from build123d import *

# Parameters (mm, degrees)
BOSS_EXTRUDE1_DEPTH     = 3
CUT_EXTRUDE1_DEPTH      = 67.166456759
CUT_EXTRUDE1_DEPTH_BACK = 67.166456759
SKETCH2_W               = 4.5
SKETCH2_H               = 4
SKETCH2_W_2             = 1.5
SKETCH2_W_3             = 6
VARFILLET1_START        = -1
VARFILLET1_DEPTH        = 5
BOSS_EXTRUDE2_START     = 1.8
SKETCH3_W               = 0.749988865
SKETCH3_H               = 2
SKETCH3_H_2             = 1.495913235
BOSS_EXTRUDE2_DEPTH     = 1.8


with BuildPart() as part:
    # Sketch1 → Boss-Extrude1 (new body)
    with BuildSketch(Plane.XY):
        with BuildLine():
            ThreePointArc((-34.616983549, 0), (-33.558491775, 0.00446614), (-32.5, 0))
            Line((-32.5, 0), (-32.5, 12))
            Line((-32.5, 12), (-48.75, 12))
            ThreePointArc((-48.75, 12), (-58.482695155, 8.177087189), (-65, 0))
            Line((-65, 0), (-34.616983549, 0))
        make_face()
        with BuildLine():
            ThreePointArc((-65, -4), (-49.931106105, -1.068651698), (-34.616983549, 0))
            Line((-34.616983549, 0), (-65, 0))
            Line((-65, 0), (-65, -4))
        make_face()
        with BuildLine():
            Line((-30.383016451, 0), (0, 0))
            ThreePointArc((0, 0), (-6.517304845, 8.177087189), (-16.25, 12))
            Line((-16.25, 12), (-32.5, 12))
            Line((-32.5, 12), (-32.5, 0))
            ThreePointArc((-32.5, 0), (-31.441508225, 0.00446614), (-30.383016451, 0))
        make_face()
        with BuildLine():
            Line((0, -4), (0, 0))
            Line((0, 0), (-30.383016451, 0))
            ThreePointArc((-30.383016451, 0), (-15.068893895, -1.068651698), (0, -4))
        make_face()
    extrude(amount=BOSS_EXTRUDE1_DEPTH)

    # Sketch2 → Cut-Extrude1 (cut, two sides: drawn at the far end of the back side and taken through both)
    with BuildSketch(Plane.XY.offset(3).offset(-CUT_EXTRUDE1_DEPTH_BACK)):
        with Locations((-34.75, 4)):
            Rectangle(SKETCH2_W, SKETCH2_H)
        with Locations((-31.75, 4)):
            Rectangle(SKETCH2_W_2, SKETCH2_H)
        with Locations((-28, 4)):
            Rectangle(SKETCH2_W_3, SKETCH2_H)
    extrude(amount=CUT_EXTRUDE1_DEPTH + CUT_EXTRUDE1_DEPTH_BACK, mode=Mode.SUBTRACT)

    # VarFillet1: read off the stored shape, not the designer's step
    # VarFillet1 outline → VarFillet1 (cut)
    with BuildSketch(Plane.XY.offset(VARFILLET1_START)):
        with BuildLine():
            ThreePointArc((-65, -4), (-64.073975757, -3.763989534), (-63.146180361, -3.535040754))
            add(Edge.make_bspline(
                [(-63.146180361, -3.535040754), (-65, -3.98501659), (-65, -2.07736738)],
                knots=[0, 0, 0, 1, 1, 1], degree=2, weights=[1, 0.61811012, 1]))
            Line((-65, -2.07736738), (-65, -4))
        make_face()
        with BuildLine():
            add(Edge.make_bspline(
                [(-0.135016199, 0.302883516), (0, 0.006564618), (0, -0.31906441)],
                knots=[0, 0, 0, 1, 1, 1], degree=2, weights=[1, 0.977238252, 1]))
            Line((0, -0.31906441), (0, 0))
            ThreePointArc((0, 0), (-0.066886569, 0.151718817), (-0.135016199, 0.302883516))
        make_face()
        with BuildLine():
            add(Edge.make_bspline(
                [(0, -2.07736738), (0, -3.98501659), (-1.853819639, -3.535040754)],
                knots=[0, 0, 0, 1, 1, 1], degree=2, weights=[1, 0.61811012, 1]))
            ThreePointArc((-1.853819639, -3.535040754), (-0.926024243, -3.763989534), (0, -4))
            Line((0, -4), (0, -2.07736738))
        make_face()
        with BuildLine():
            Line((-65, 0), (-65, -0.31906441))
            add(Edge.make_bspline(
                [(-65, -0.31906441), (-65, 0.006564618), (-64.864983801, 0.302883516)],
                knots=[0, 0, 0, 1, 1, 1], degree=2, weights=[1, 0.977238252, 1]))
            ThreePointArc((-64.864983801, 0.302883516), (-64.933113431, 0.151718817), (-65, 0))
        make_face()
    extrude(amount=VARFILLET1_DEPTH, mode=Mode.SUBTRACT)

    # Sketch3 → Boss-Extrude2 (add)
    with BuildSketch(Plane(origin=(0, 0, 0), x_dir=(-1, 0, 0), z_dir=(0, 0, -1)).offset(BOSS_EXTRUDE2_START)):
        with Locations((32.125005567, 11)):
            Rectangle(SKETCH3_W, SKETCH3_H)
        with Locations((32.874994433, 11)):
            Rectangle(SKETCH3_W, SKETCH3_H)
        with Locations((32.125005567, 0.752043383)):
            Rectangle(SKETCH3_W, SKETCH3_H_2)
        with BuildLine():
            Line((32.5, 0.004086765), (32.5, 0))
            ThreePointArc((32.5, 0), (32.874991378, 0.002603923), (33.249988865, 0.004086765))
            Line((33.249988865, 0.004086765), (33.249988865, 1.5))
            Line((33.249988865, 1.5), (32.5, 1.5))
            Line((32.5, 1.5), (32.5, 0.004086765))
        make_face()
    extrude(amount=-BOSS_EXTRUDE2_DEPTH)


solid = part.part
Here's how the part is built. I have some questions about the finished solid (model axes, mm). A direction names the side the tool comes from. Coordinates: 2 decimals unless noted, no trailing zeros. Loops run counter-clockwise (first coordinate to the right, second up) from the corner with the lowest first, then second, coordinate; pieces in that order, holes last. Notation, with made-up numbers: (-6, 22) -> (10, 22) arc R17 cw to (10, 44) -> close; hole circle Ø2 at (49.25, -19). An arc over 180 degrees is marked (long way). Use one line per item in the form item = value. Start each with the question number.
(1) On a 3-axis mill with a long thin cutter (end or side, diameter ignored), from which of +Z, -Z, +X, -X, +Y, -Y can I reach the whole of each face in a straight line? I mean faces 4 (the face through (-32, 10, -1)), 5 (the face through (-31.75, 1, -1)), 6 (the face through (-33, 8, 3)), 7 (the face through (-33.25, 11, -1)), 8 (the face through (-31, 2, 1)). Say none if no direction works.
(2) Please list where these lines run through material, in increasing order: line 1 along Z through (x, y) = (-46.5, 2); line 2 along X through (y, z) = (4.5, 2.05); line 3 along X through (y, z) = (1.25, -0.3).
(3) If we section it at D-D (x = -42): Please give me the cut outline in (y, z), then the cut area to 3 significant figures.
(4) Will these pins go through, and if not, where does the flat tip stop? pin 1 (8 mm diameter, centred on x = -20.5, y = 4.5, fed in from -Z); pin 2 (1.2 mm diameter, centred on x = -32.5, z = -0.5, fed in from -Y); pin 3 (1.5 mm diameter, centred on x = -17, z = 2, fed in from -Y).
(5) We'd pull the mould along Y, two halves only. Please class faces 1 (the face through (-32, 1, -1.8)), 2 (the face through (-33, 1.5, -1)), 3 (the face through (-32, 12, 1)): pulls with the +Y half, pulls with the -Y half, needs draft (parallel to the pull), parting line crosses it, or undercut.
(6) If we section it at C-C (y = -1.25): Please give me the cut outline in (x, z).
(7) If we section it at B-B (y = 11.25): Please give me the cut outline in (x, z), then the cut area to 3 significant figures.
(8) If we section it at A-A (y = 2.75): Please give me the cut outline in (x, z).
Verdict:
q1.face_4 = -Z, +X, -X
q1.face_5 = -Z, +X, +Y, -Y
q1.face_6 = +Z, +X, -X, +Y, -Y
q1.face_7 = -Z, -X, +Y, -Y
q1.face_8 = +Z, -Z
q2.line_1 = 0 to 3
q2.line_2 = -62.29 to -37, -25 to -2.71
q2.line_3 = -33.25 to -31.75
q3.outline = (-0.28, 0) -> (12, 0) -> (12, 3) -> (-0.28, 3) -> close
q3.area = 36.8 mm²
q4.pin_1 = 0
q4.pin_2 = 0
q4.pin_3 = -0.92
q5.face_1 = needs draft
q5.face_2 = undercut
q5.face_3 = pulls with the +Y half
q6.outline = (-65, 0) -> (-51.25, 0) -> (-51.25, 3) -> (-65, 3) -> close; (-13.75, 0) -> (0, 0) -> (0, 3) -> (-13.75, 3) -> close
q7.outline = (-52.37, 0) -> (-33.25, 0) -> (-33.25, -1.8) -> (-31.75, -1.8) -> (-31.75, 0) -> (-12.63, 0) -> (-12.63, 3) -> (-52.37, 3) -> close
q7.area = 122 mm²
q8.outline = (-63.54, 0) -> (-37, 0) -> (-37, 3) -> (-63.54, 3) -> close; (-25, 0) -> (-1.46, 0) -> (-1.46, 3) -> (-25, 3) -> close
